Design review of the part built by this model. Coordinates are the model's own, in mm. A direction names the side the tool comes from. Coordinates: 2 decimals unless noted, no trailing zeros. Write each loop counter-clockwise with the first axis right and the second up, starting at its lowest first coordinate (ties: lowest second). Pieces come first, ordered by that corner, then holes. Notation, with made-up numbers: (25.25, 71.25) - (50.25, 71.25) arc R13 ccw to (50.25, 89.25) - close; hole circle Ø3 at (83.5, 80). An arc over 180 degrees is marked (long way). Answer as a JSON object with one key per item and string values.
Autodesk Inventor part; units mm, degrees
ref_plane "YZ Plane" through (0, 0, 0) normal (1, 0, 0) x (0, 1, 0)
ref_plane "XZ Plane" through (0, 0, 0) normal (0, 1, 0) x (-1, 0, 0)
ref_plane "XY Plane" through (0, 0, 0) normal (0, 0, 1) x (1, 0, 0)
sketch "スケッチ1" plane through (0, 0, 0) normal (0, 0, 1) x (1, 0, 0)
  circle A0 centre (0, 0) radius 1.65
  dimension "d0" = 3.3
extrude "押し出し1" add sketch "スケッチ1" along normal blind 20
sketch "スケッチ2" plane through (0, 0, 20) normal (0, 0, 1) x (1, 0, 0)
  circle A0 centre (0, 0) radius 4
  dimension "d3" = 8
extrude "押し出し2" add sketch "スケッチ2" against normal blind 2.3
chamfer "面取り1" distance 2.3 angle 45 1 edges at (-4, 0, 17.7)
thread "ねじ1"
properties part number "ネジ皿m4,20" material "鋼、高強度、低合金"
(1) Tool access review of faces 1 (the face through (0, 0, 0)), 2 (the face through (-1.216, -1.115, 8.726)): name each direction out of +Z, -Z, +X, -X, +Y, -Y from which nothing blocks a thin tool from reaching the whole face with its end or side.
Solved:
{"face 1": "-Z, +X, -X, +Y, -Y", "face 2": "-Z"}
(2) Take a section at C-C, the plane z = 14.75. Write out the cut boundary in (x, y).
Solved:
{"outline": "circle Ø3.3 at (0, 0)"}
(3) For pin 1 (4 mm diameter, centred on x = -0.5, y = -2.5, fed in from -Z); pin 2 (2 mm diameter, centred on x = 2, z = 16.5, fed in from -Y), all flat-tipped, find the tip position at first contact; note any pin that passes through.
Solved:
{"pin 1": "stops at z = 0", "pin 2": "stops at y = -1.31"}
(4) To check wall thickness, follow line 1 (Z direction, x = -2, y = 1.75); line 2 (Z direction, x = -0.5, y = 2.25); line 3 (Y direction, x = 1.5, z = 8.5). State the ranges of each line that lie inside material, in increasing order. Write a range as from..to.
Solved:
{"line 1": "z = 18.66..20", "line 2": "z = 18.3..20", "line 3": "y = -0.69..0.69"}
